Design review of the part built by this model. Coordinates are the model's own, in mm. A direction names the side the tool comes from. Coordinates: 2 decimals unless noted, no trailing zeros. Order: outer loops, then holes, each group sorted by start corner. A loop starts at its lowest first (then second) coordinate and runs counter-clockwise, first axis right, second up. Notation, with made-up numbers: M 77.5,-40 L 124.5,-40 A25 cw 124.5,-24 Z; hole C 83.5,62.25 d3. An arc over 180 degrees is marked long. Answer in a Markdown table with one row per item.
from build123d import *

# Parameters (mm, degrees)
CYLINDER048_R          = 4.7
CYLINDER048_DEPTH      = 100
CYLINDER048_ROLL_ANGLE = 90
CYLINDER045_R          = 1.8
CYLINDER045_DEPTH      = 20
CYLINDER044_R          = 3
CYLINDER044_DEPTH      = 10
CYLINDER042_R          = 1.8
CYLINDER042_DEPTH      = 20
CYLINDER041_R          = 3
CYLINDER041_DEPTH      = 10
CYLINDER034_R          = 3
CYLINDER034_DEPTH      = 10
CYLINDER033_R          = 3
CYLINDER033_DEPTH      = 10
CYLINDER031_R          = 1.8
CYLINDER031_DEPTH      = 20
CYLINDER032_R          = 1.8
CYLINDER032_DEPTH      = 20
CYLINDER029_R          = 7.8
CYLINDER029_DEPTH      = 24.85
CYLINDER029_ROLL_ANGLE = 90
CYLINDER030_R          = 4.4
CYLINDER030_DEPTH      = 76.1
CYLINDER030_ROLL_ANGLE = 90
CYLINDER028_R          = 7.8
CYLINDER028_DEPTH      = 24.85
CYLINDER028_ROLL_ANGLE = 90
BOX011_W               = 23
BOX011_H               = 76.1
BOX011_DEPTH           = 8
FILLET003002_R         = 1


with BuildPart() as cylinder048:
    # Cylinder048 → Cylinder048 (new body)
    with BuildSketch(Plane.XY):
        Circle(CYLINDER048_R)
    extrude(amount=CYLINDER048_DEPTH)


with BuildPart() as cylinder048_1:
    # Cylinder048 roll: moved
    add(cylinder048.part.rotate(Axis((0, 0, 0), (1, 0, 0)), CYLINDER048_ROLL_ANGLE))


with BuildPart() as cylinder048_2:
    # Cylinder048 placement: moved
    add(cylinder048_1.part.moved(Location((12, 79, 0))))


with BuildPart() as cilindro030:
    # Cylinder045 → Cylinder045 (new body)
    with BuildSketch(Plane(origin=(19, 5, -10), x_dir=(1, 0, 0), z_dir=(0, 0, 1))):
        Circle(CYLINDER045_R)
    extrude(amount=CYLINDER045_DEPTH)


with BuildPart() as cilindro029:
    # Cylinder044 → Cylinder044 (new body)
    with BuildSketch(Plane(origin=(19, 5, -15), x_dir=(1, 0, 0), z_dir=(0, 0, 1))):
        Circle(CYLINDER044_R)
    extrude(amount=CYLINDER044_DEPTH)


with BuildPart() as cilindro027:
    # Cylinder042 → Cylinder042 (new body)
    with BuildSketch(Plane(origin=(19, 72, -10), x_dir=(1, 0, 0), z_dir=(0, 0, 1))):
        Circle(CYLINDER042_R)
    extrude(amount=CYLINDER042_DEPTH)


with BuildPart() as cilindro026:
    # Cylinder041 → Cylinder041 (new body)
    with BuildSketch(Plane(origin=(19, 72, -15), x_dir=(1, 0, 0), z_dir=(0, 0, 1))):
        Circle(CYLINDER041_R)
    extrude(amount=CYLINDER041_DEPTH)


with BuildPart() as cilindro019:
    # Cylinder034 → Cylinder034 (new body)
    with BuildSketch(Plane(origin=(5, 72, -15), x_dir=(1, 0, 0), z_dir=(0, 0, 1))):
        Circle(CYLINDER034_R)
    extrude(amount=CYLINDER034_DEPTH)


with BuildPart() as cilindro018:
    # Cylinder033 → Cylinder033 (new body)
    with BuildSketch(Plane(origin=(5, 5, -15), x_dir=(1, 0, 0), z_dir=(0, 0, 1))):
        Circle(CYLINDER033_R)
    extrude(amount=CYLINDER033_DEPTH)


with BuildPart() as cilindro016:
    # Cylinder031 → Cylinder031 (new body)
    with BuildSketch(Plane(origin=(5, 5, -10), x_dir=(1, 0, 0), z_dir=(0, 0, 1))):
        Circle(CYLINDER031_R)
    extrude(amount=CYLINDER031_DEPTH)


with BuildPart() as cilindro017:
    # Cylinder032 → Cylinder032 (new body)
    with BuildSketch(Plane(origin=(5, 72, -10), x_dir=(1, 0, 0), z_dir=(0, 0, 1))):
        Circle(CYLINDER032_R)
    extrude(amount=CYLINDER032_DEPTH)


with BuildPart() as cylinder029:
    # Cylinder029 → Cylinder029 (new body)
    with BuildSketch(Plane.XY):
        Circle(CYLINDER029_R)
    extrude(amount=CYLINDER029_DEPTH)


with BuildPart() as cylinder029_1:
    # Cylinder029 roll: moved
    add(cylinder029.part.rotate(Axis((0, 0, 0), (1, 0, 0)), CYLINDER029_ROLL_ANGLE))


with BuildPart() as cylinder029_2:
    # Cylinder029 placement: moved
    add(cylinder029_1.part.moved(Location((12.25, 68.1, 0))))


with BuildPart() as cylinder030:
    # Cylinder030 → Cylinder030 (new body)
    with BuildSketch(Plane.XY):
        Circle(CYLINDER030_R)
    extrude(amount=CYLINDER030_DEPTH)


with BuildPart() as cylinder030_1:
    # Cylinder030 roll: moved
    add(cylinder030.part.rotate(Axis((0, 0, 0), (1, 0, 0)), CYLINDER030_ROLL_ANGLE))


with BuildPart() as cylinder030_2:
    # Cylinder030 placement: moved
    add(cylinder030_1.part.moved(Location((12.25, 76.1, 0))))


with BuildPart() as cylinder028:
    # Cylinder028 → Cylinder028 (new body)
    with BuildSketch(Plane.XY):
        Circle(CYLINDER028_R)
    extrude(amount=CYLINDER028_DEPTH)


with BuildPart() as cylinder028_1:
    # Cylinder028 roll: moved
    add(cylinder028.part.rotate(Axis((0, 0, 0), (1, 0, 0)), CYLINDER028_ROLL_ANGLE))


with BuildPart() as cylinder028_2:
    # Cylinder028 placement: moved
    add(cylinder028_1.part.moved(Location((12.25, 35.55, 0))))


with BuildPart() as obj1:
    # Box011 → Box011 (new body)
    with BuildSketch(Plane.XY.offset(-8)):
        with Locations((11.5, 38.05)):
            Rectangle(BOX011_W, BOX011_H)
    extrude(amount=BOX011_DEPTH)

    # Cut010035003006: cut Cylinder028
    add(cylinder028_2.part, mode=Mode.SUBTRACT)

    # Cut010035003007: cut Cylinder030
    add(cylinder030_2.part, mode=Mode.SUBTRACT)

    # Cut010035003008: cut Cylinder029
    add(cylinder029_2.part, mode=Mode.SUBTRACT)

    # Cut010035003009: cut Cilindro017
    add(cilindro017.part, mode=Mode.SUBTRACT)

    # Cut010035003010: cut Cilindro016
    add(cilindro016.part, mode=Mode.SUBTRACT)

    # Fillet003002
    fillet003002_edges = [obj1.edges().sort_by_distance(p)[0] for p in [
        (0, 0, -4),
        (0, 76.1, -4),
        (23, 0, -4),
        (23, 76.1, -4),
    ]]
    fillet(fillet003002_edges, radius=FILLET003002_R)

    # Cut010035003011: cut Cilindro018
    add(cilindro018.part, mode=Mode.SUBTRACT)

    # Cut010035003012: cut Cilindro019
    add(cilindro019.part, mode=Mode.SUBTRACT)

    # Cut010035003022: cut Cilindro026
    add(cilindro026.part, mode=Mode.SUBTRACT)

    # Cut010035003023: cut Cilindro027
    add(cilindro027.part, mode=Mode.SUBTRACT)

    # Cut010035003026: cut Cilindro029
    add(cilindro029.part, mode=Mode.SUBTRACT)

    # Cut010035003027: cut Cilindro030
    add(cilindro030.part, mode=Mode.SUBTRACT)

    # Cut010035003032: cut Cylinder048
    add(cylinder048_2.part, mode=Mode.SUBTRACT)


solid = obj1.part
(1) Add section C-C, the plane x = 5.75. Give the boundary of the cut face in (y, z), and give its area (3 significant figures).
Return value:
| item | result |
|---|---|
| outline | M 0,-8 L 2.1,-8 L 2.1,-5 L 3.36,-5 L 3.36,0 L 0,0 Z; M 6.64,-5 L 7.9,-5 L 7.9,-8 L 69.1,-8 L 69.1,-5 L 70.36,-5 L 70.36,0 L 68.1,0 L 68.1,-4.31 L 43.25,-4.31 L 43.25,0 L 35.55,0 L 35.55,-4.31 L 10.7,-4.31 L 10.7,0 L 6.64,0 Z; M 73.64,-5 L 74.9,-5 L 74.9,-8 L 76.1,-8 L 76.1,0 L 73.64,0 Z |
| area | 327 mm2 |
(2) Insertion check: pin 1 Ø3 at (x, y) = (19, 72.5) entering from -Z; pin 2 Ø8 at (x, y) = (19, 5) entering from -Z. Each pin has a flat end and moves straight along its axis. Give the tip position at first contact, or say it passes through.
Return value:
| item | result |
|---|---|
| pin 1 | stops at z = -5 |
| pin 2 | stops at z = -8 |
(3) Draft analysis for pull direction X (two halves, no side actions). For faces 1 (the flat face through (11, 39, -8)), 2 (the flat face through (23, 38, -4)), 3 (the cylindrical face through (18.61, 3.243, -2.535)), state which applies: pulls with the +X half, pulls with the -X half, needs draft (parallel to the pull), parting line crosses it, or undercut.
Return value:
| item | result |
|---|---|
| face 1 | needs draft |
| face 2 | pulls with the +X half |
| face 3 | undercut |
(4) Add section D-D, the plane z = -5.75. Give the boundary of the cut face in (x, y).
Return value:
| item | result |
|---|---|
| outline | M 0,1 A1 ccw 1,0 L 22,0 A1 ccw 23,1 L 23,75.1 A1 ccw 22,76.1 L 1,76.1 A1 ccw 0,75.1 Z; hole C 5,5 d6; hole C 5,72 d6; hole M 6.98,10.7 L 17.52,10.7 L 17.52,35.55 L 6.98,35.55 Z; hole M 6.98,43.25 L 17.52,43.25 L 17.52,68.1 L 6.98,68.1 Z; hole C 19,5 d6; hole C 19,72 d6 |
(5) Add section B-B, the plane z = -1. Give the number of separate pieces and of enclosed holes in the cut face, and give its area (3 significant figures).
Return value:
| item | result |
|---|---|
| separate pieces | 2 |
| enclosed holes | 4 |
| area | 697 mm2 |
(6) For line 1 along X through (y, z) = (5, -6.9); line 2 along Y through (x, z) = (19, -1.85); line 3 along Y through (x, z) = (8.75, -5.25), list the stretches that pass through material, from the lowest coordinate up. Write a range as from..to.
Return value:
| item | result |
|---|---|
| line 1 | x = 0..2, 8..16, 22..23 |
| line 2 | y = 0..3.2, 6.8..10.7, 35.55..43.25, 68.1..70.2, 73.8..76.1 |
| line 3 | y = 0..10.7, 35.55..43.25, 68.1..76.1 |
(7) For faces 4 (the cylindrical face through (4.35, 69.07, -6.52)), 5 (the cylindrical face through (5.831, 3.403, -2.535)), 6 (the flat face through (12, 35.55, -5)), list the 3-axis set-ups (+Z, -Z, +X, -X, +Y, -Y) from which the entire face can be reached by the end or side of a thin tool; tool diameter is ignored.
Return value:
| item | result |
|---|---|
| face 4 | -Z |
| face 5 | +Z, -Z |
| face 6 | +Z |
(8) Add section A-A, the plane y = 5. Give the boundary of the cut face in (x, z).
Return value:
| item | result |
|---|---|
| outline | M 0,-8 L 2,-8 L 2,-5 L 3.2,-5 L 3.2,0 L 0,0 Z; M 6.8,-5 L 8,-5 L 8,-8 L 16,-8 L 16,-5 L 17.2,-5 L 17.2,0 L 16.7,0 A4.7 cw 7.3,0 L 6.8,0 Z; M 20.8,-5 L 22,-5 L 22,-8 L 23,-8 L 23,0 L 20.8,0 Z |
